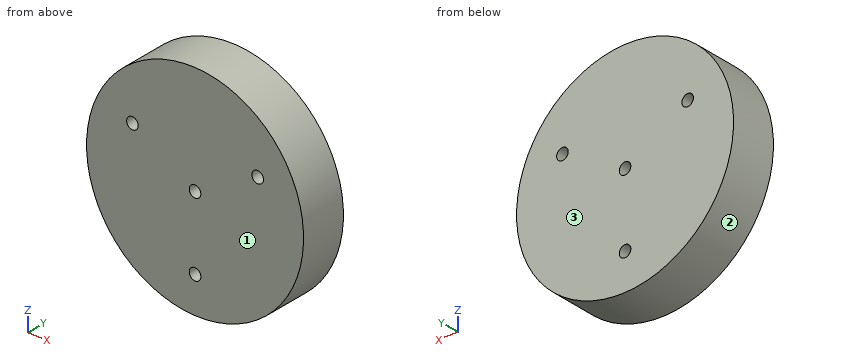
```python
from build123d import *

# Parameters (mm, degrees)
SKETCH1_R           = 75
BOSS_EXTRUDE1_DEPTH = 32
SKETCH2_R           = 4
CUT_EXTRUDE1_DEPTH  = 111.788086002
CIRPATTERN1_COUNT   = 3
SKETCH3_R           = 4
CUT_EXTRUDE2_DEPTH  = 111.788086002


with BuildPart() as part:
    # Sketch1 → Boss-Extrude1 (new body)
    with BuildSketch(Plane(origin=(0, 0, 0), x_dir=(1, 0, 0), z_dir=(0, 1, 0))):
        with Locations(Location((0, 0, 0), (0, 0, 270))):
            Circle(SKETCH1_R)
    extrude(amount=BOSS_EXTRUDE1_DEPTH)

    # Sketch2 → Cut-Extrude1 (cut, through all)
    with BuildSketch(Plane(origin=(0, 32, 0), x_dir=(1, 0, 0), z_dir=(0, 1, 0))):
        with Locations(Location((0, 50, 0), (0, 0, 270))):
            Circle(SKETCH2_R)
    cut_extrude1 = extrude(amount=-CUT_EXTRUDE1_DEPTH, mode=Mode.SUBTRACT)

    # CirPattern1: Cut-Extrude1 ×3 about axis
    cirpattern1_axis = Axis((0, 0, 0), (0, 1, 0))
    for i in range(1, CIRPATTERN1_COUNT):
        add(cut_extrude1.rotate(cirpattern1_axis, i * 360 / CIRPATTERN1_COUNT), mode=Mode.SUBTRACT)

    # Sketch3 → Cut-Extrude2 (cut, through all)
    with BuildSketch(Plane(origin=(0, 32, 0), x_dir=(1, 0, 0), z_dir=(0, 1, 0))):
        with Locations(Location((0, 0, 0), (0, 0, 270))):
            Circle(SKETCH3_R)
    extrude(amount=-CUT_EXTRUDE2_DEPTH, mode=Mode.SUBTRACT)


solid = part.part
```
Source: CAD feature listing. Evaluate the final solid. Frame: model axes, mm. Face numbers are marked on the shaded views. Coordinates: 2 decimals unless noted, no trailing zeros. Order: outer loops, then holes, each group sorted by start corner. A loop starts at its lowest first (then second) coordinate and runs counter-clockwise, first axis right, second up. Notation, with made-up numbers: M -5.75,10.25 L 40.25,10.25 A21 ccw 40.25,44.25 Z; hole C 46.25,10 d10. An arc over 180 degrees is marked long. Write each question's results on one line, items separated by ' | '. Start each with the question number.
1) Section query A-A (z = 0). Return the cut outline in (x, y).
2) Section query D-D (z = -50). Return the cut outline in (x, y), plus the area to 3 significant figures.
3) Contact query for flat-ended pins moving along their axis: pin 1 Ø2 at (x, y) = (-26, 19) entering from -Z; pin 2 Ø1 at (x, y) = (27, 11) entering from +Z; pin 3 Ø13 at (x, z) = (0, 0) entering from -Y; pin 4 Ø8 at (y, z) = (15.5, 39) entering from +X. Output: stop coordinate, or through.
4) Section query B-B (x = 0). Return the cut outline in (y, z), plus the area to 3 significant figures.
5) Section query C-C (y = 11). Return the cut outline in (x, z).
6) Line query: line 1 (X direction, y = 7.5, z = 25); line 2 (X direction, y = 22, z = 0); line 3 (Z direction, x = -67, y = 17). Output: solid intervals per line, ascending. Write a range as from..to.
7) Draft query along Y for the marked faces 1, 2 and 3. Return one class per face: released by +Y, released by -Y, zero draft, split by the parting line, or undercut.
Answers:
1) outline: M -75,0 L -4,0 L -4,32 L -75,32 Z; M 4,0 L 75,0 L 75,32 L 4,32 Z
2) outline: M -55.9,0 L -4,0 L -4,32 L -55.9,32 Z; M 4,0 L 55.9,0 L 55.9,32 L 4,32 Z | area: 3,320 mm^2
3) pin 1: stops at z = -70.71 | pin 2: stops at z = 70.16 | pin 3: stops at y = 0 | pin 4: stops at x = 66.33
4) outline: M 0,-75 L 32,-75 L 32,-54 L 0,-54 Z; M 0,-46 L 32,-46 L 32,-4 L 0,-4 Z; M 0,4 L 32,4 L 32,75 L 0,75 Z | area: 4,290 mm^2
5) outline: C 0,0 d150; hole C -43.3,25 d8; hole C 0,-50 d8; hole C 0,0 d8; hole C 43.3,25 d8
6) line 1: x = -70.71..-47.3, -39.3..39.3, 47.3..70.71 | line 2: x = -75..-4, 4..75 | line 3: z = -33.7..33.7
7) face 1: released by -Y | face 2: zero draft | face 3: released by +Y
